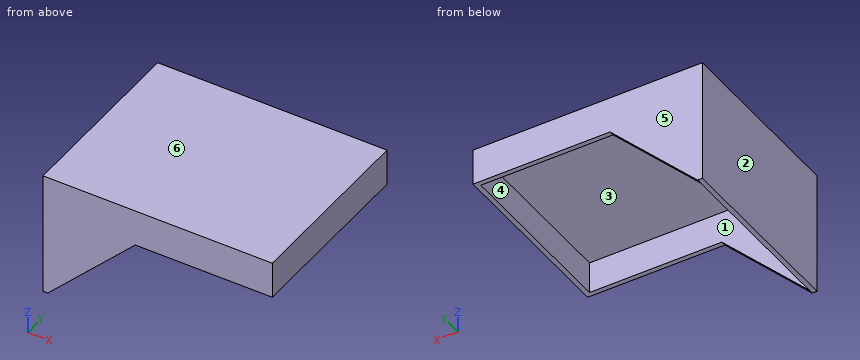
Autodesk Inventor part; units mm, degrees
ref_plane "YZ Plane" through (0, 0, 0) normal (1, 0, 0) x (0, 1, 0)
ref_plane "XZ Plane" through (0, 0, 0) normal (0, 1, 0) x (-1, 0, 0)
ref_plane "XY Plane" through (0, 0, 0) normal (0, 0, 1) x (1, 0, 0)
sketch "Эскиз1" plane through (0, 0, 0) normal (0, 0, 1) x (1, 0, 0)
  line L0 (29.9444, -74.6554) -> (-27.0756, -74.6554)
  line L1 (29.9444, 31.7946) -> (29.9444, -74.6554)
  line L2 (-27.0756, 31.7946) -> (29.9444, 31.7946)
  line L3 (-27.0756, -74.6554) -> (-27.0756, 31.7946)
  circle A0 centre (-22.2656, 27.6646) radius 2
  circle A1 centre (-22.2656, -70.5254) radius 2
  circle A2 centre (25.1344, -70.5254) radius 2
  circle A3 centre (25.1344, 27.6646) radius 2
  line L4 (-29.0756, 55) -> (29.0756, 55)
  line L5 (29.0756, 55) -> (29.0756, -55)
  line L6 (29.0756, -55) -> (-29.0756, -55)
  line L7 (-29.0756, -55) -> (-29.0756, 55)
  line L8 (-29.0756, 55) -> (29.0756, -55) construction
  line L9 (29.0756, 55) -> (-29.0756, -55) construction
  line L10 (-32.0756, 58) -> (32.0756, 58)
  line L11 (32.0756, 58) -> (32.0756, -58)
  line L12 (32.0756, -58) -> (-32.0756, -58)
  line L13 (-32.0756, -58) -> (-32.0756, 58)
  line L14 (29.0756, 55) -> (109.0756, 55)
  line L15 (109.0756, 55) -> (109.0756, -55)
  line L16 (109.0756, -55) -> (29.0756, -55)
  line L17 (32.0756, -58) -> (112.0756, -58)
  line L18 (112.0756, -58) -> (112.0756, 58)
  line L19 (112.0756, 58) -> (32.0756, 58)
  point P0 (0, 0)
  dimension "d0" = 110
  dimension "d1" = 2
  dimension "d2" = 3
  dimension "d3" = 80
  dimension "d4" = 80
extrude "Выдавливание1" add sketch "Эскиз1" along normal blind 3 contours L12 L3 L6 L16 L1 | L1 L16 L11 L12 | L12 L13 L10 L11 L14 L4 L7 L6 L3 | L16 L5 L2 L1 | L1 L2 L5 L14 L11 L16 | L11 L16 L15 L14 L19 L18 L17 | L6 L7 L4 L5 L2 L3 | L3 L2 L5 L6 | L11 L14 L15 L16 | A0 | A3
sketch "Эскиз2" plane through (0, 0, 0) normal (0, 0, -1) x (-1, 0, 0)
  line L0 (-112.0756, -58) -> (-112.0756, 58)
  line L1 (32.0756, -58) -> (-112.0756, -58)
  line L2 (32.0756, 58) -> (32.0756, -58)
  line L3 (-112.0756, 58) -> (32.0756, 58)
  line L4 (-109.0756, -55) -> (-109.0756, 55)
  line L5 (-109.0756, 55) -> (29.0756, 55)
  line L6 (29.0756, 55) -> (29.0756, -55)
  line L7 (29.0756, -55) -> (-109.0756, -55)
  point P0 (0, 0)
  dimension "d7" = 3
extrude "Выдавливание2" add sketch "Эскиз2" along normal blind 75
sketch "Эскиз3" plane through (-32.0756, 58, 3) normal (0, 1, 0) x (1, 0, 0)
  line L0 (3, 3) -> (3, 78)
  line L1 (3, 78) -> (78, 3)
  line L2 (3, 3) -> (141.1512, 3)
  line L3 (0, 78) -> (0, 0)
  line L4 (144.1512, 0) -> (0, 0)
  line L5 (144.1512, 78) -> (144.1512, 0)
  line L6 (0, 78) -> (144.1512, 78)
  line L7 (141.1512, 3) -> (141.1512, 78)
  line L8 (141.1512, 3) -> (144.1512, 3)
  line L9 (144.1512, 78) -> (144.1512, 0)
  line L10 (144.1512, 3) -> (144.1512, 18)
  line L11 (144.1512, 0) -> (144.1512, 78)
  line L12 (144.1512, 18) -> (63, 18)
  line L13 (135.5856, 23) -> (56.5656, 23)
  line L14 (58, 23) -> (144.1512, 23)
  point P0 (32.0756, 3)
  point P1 (78, 3)
  point P2 (3, 78)
  point P3 (144.1512, 3)
  point P4 (144.1512, 18)
  point P5 (58, 23)
  point P6 (134.1512, 23)
  dimension "d10" = 45
  dimension "d13" = 15
extrude "Выдавливание3" cut sketch "Эскиз3" against normal up to surface (116 mm away) contours L6 L7 L14 L13 L1 | L6 L5 L14 L7
sketch "Эскиз4" plane through (-32.0756, -58, 3) normal (-1, 0, 0) x (0, 0, 1)
  line L0 (-78, 116) -> (-78, 113)
  line L1 (-78, 116) -> (-72, 116)
  line L2 (-23, 116) -> (-78, 116)
  line L3 (-72, 116) -> (-72, 0)
  line L4 (-78, 0) -> (0, 0)
  point P0 (-3, 58)
  point P1 (-18, 116)
  point P2 (-3, 116)
  dimension "d14" = 6
sketch "Эскиз5" plane through (112.0756, -58, 3) normal (1, 0, 0) x (0, 0, -1)
  line L0 (78, 116) -> (0, 116)
  line L1 (23, 116) -> (0, 116)
  line L2 (11.5, 116) -> (11.5, 0)
  line L3 (78, 0) -> (0, 0)
  point P0 (3, 58)
properties part number "LPS_base"
Geometry check sheet. Reference: the model listing, model coordinates, mm. Face numbers are marked on the shaded views. A direction names the side the tool comes from. Round coordinates to 2 decimals unless told otherwise and drop trailing zeros. Loops run counter-clockwise (first coordinate to the right, second up) from the corner with the lowest first, then second, coordinate; pieces in that order, holes last. Notation, with made-up numbers: (20, -29) -> (41, -29) arc R12 cw to (41, -21) -> close; hole circle Ø7 at (50.25, 49). An arc over 180 degrees is marked (long way). Answer as a JSON object with one key per item and string values. Group by question number.
Item 1: Set-up check for the marked faces 1 and 2: record each of +Z, -Z, +X, -X, +Y, -Y from which the full face is reachable in a straight line by a thin tool's end or side.
Item 2: Depth check by flat-ended pin: pin 1 Ø5 at (x, y) = (89, -6.5) entering from -Z; pin 2 Ø8 at (x, z) = (48, -22) entering from -Y; pin 3 Ø10 at (y, z) = (-9.5, -36) entering from +X. Enter the tip coordinate at first touch or a pass-through.
Item 3: Cross-section at C-C, the plane y = 50. Record the cut outline in (x, z), plus the area to 3 significant figures.
Item 4: Cross-section at A-A, the plane z = -14.5. Record the cut outline in (x, y).
Item 5: Cross-section at B-B, the plane x = 43. Record the cut outline in (y, z).
Item 6: Thickness scan on line 1 along Y through (x, z) = (-13, -38); line 2 along X through (y, z) = (50, -6.5); line 3 along X through (y, z) = (4, -51). Record the ranges inside material, lowest first.
Item 7: Release check for a two-part mould opening along Y. For the marked faces 3, 4, 5 and 6 record: pulls with the +Y half, pulls with the -Y half, needs draft (parallel to the pull), parting line crosses it, or undercut.
Determined:
{
 "1": {"face 1": "-Z", "face 2": "+Z, -Z, -X, +Y, -Y"},
 "2": {"pin 1": "stops at z = 0", "pin 2": "stops at y = -58", "pin 3": "stops at x = -29.08"},
 "3": {"outline": "(-32.08, -75) -> (-29.08, -75) -> (-29.08, 0) -> (109.08, 0) -> (109.08, -20) -> (112.08, -20) -> (112.08, 3) -> (-32.08, 3) -> close", "area": "717 mm²"},
 "4": {"outline": "(-32.08, -58) -> (112.08, -58) -> (112.08, 58) -> (-32.08, 58) -> close; hole (-29.08, -55) -> (109.08, -55) -> (109.08, 55) -> (-29.08, 55) -> close"},
 "5": {"outline": "(-58, -20) -> (-55, -20) -> (-55, 0) -> (55, 0) -> (55, -20) -> (58, -20) -> (58, 3) -> (-58, 3) -> close"},
 "6": {"line 1": "y = -58 to -55, 55 to 58", "line 2": "x = -32.08 to -29.08, 109.08 to 112.08", "line 3": "x = -32.08 to -29.08"},
 "7": {"face 3": "undercut", "face 4": "undercut", "face 5": "pulls with the +Y half", "face 6": "needs draft"}
}
